Autodesk Inventor part; units mm, degrees
ref_plane "YZ Plane" through (0, 0, 0) normal (1, 0, 0) x (0, 1, 0)
ref_plane "XZ Plane" through (0, 0, 0) normal (0, 1, 0) x (-1, 0, 0)
ref_plane "XY Plane" through (0, 0, 0) normal (0, 0, 1) x (1, 0, 0)
sketch "Sketch_1" plane through (0, 0, 0) normal (0, 0, 1) x (1, 0, 0)
  line L0 (-57.15, 38.1) -> (-57.15, 0)
  line L1 (-57.15, 0) -> (57.15, 0)
  line L2 (57.15, 0) -> (57.15, 114.3)
  line L3 (57.15, 114.3) -> (19.05, 114.3)
  line L4 (19.05, 114.3) -> (-57.15, 38.1)
  circle A0 centre (38.1, 19.05) radius 4.1656
  circle A1 centre (38.1, 57.15) radius 4.1656
  circle A2 centre (38.1, 95.25) radius 4.1656
  circle A3 centre (0, 19.05) radius 4.1656
  circle A4 centre (0, 57.15) radius 4.1656
  circle A5 centre (-38.1, 19.05) radius 4.1656
extrude "Extrusion1" add sketch "Sketch_1" along normal mid plane 6.35
properties part number "4461"
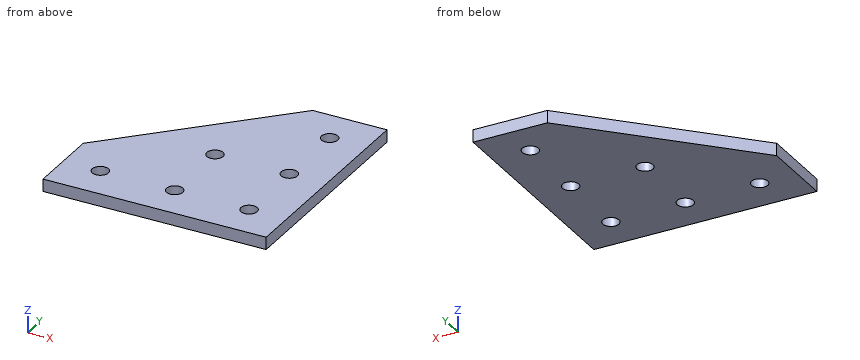
The model under review builds one solid part; all positions refer to its coordinate system, in mm. Coordinates: 2 decimals unless noted, no trailing zeros. Loops run counter-clockwise (first coordinate to the right, second up) from the corner with the lowest first, then second, coordinate; pieces in that order, holes last.
(1) Consider section C-C, the plane z = -1. Give the boundary of the cut face in (x, y).
Determined:
outline: (-57.15, 0) - (57.15, 0) - (57.15, 114.3) - (19.05, 114.3) - (-57.15, 38.1) - close; hole circle Ø8.33 at (-38.1, 19.05); hole circle Ø8.33 at (0, 19.05); hole circle Ø8.33 at (0, 57.15); hole circle Ø8.33 at (38.1, 19.05); hole circle Ø8.33 at (38.1, 57.15); hole circle Ø8.33 at (38.1, 95.25)
(2) Wall thickness on L1, parallel to Y at x = 38.1, z = -2; L2, parallel to X at y = 71, z = 0; L3, parallel to Y at x = 10, z = 2.5: over which ranges is each line inside the solid? List them lowest first.
Determined:
L1: y = 0 to 14.88, 23.22 to 52.98, 61.32 to 91.08, 99.42 to 114.3
L2: x = -24.25 to 57.15
L3: y = 0 to 105.25
(3) Consider section D-D, the plane x = -38.1. Give the boundary of the cut face in (y, z) (3 decimals).
Determined:
outline: (0, -3.175) - (14.884, -3.175) - (14.884, 3.175) - (0, 3.175) - close; (23.216, -3.175) - (57.15, -3.175) - (57.15, 3.175) - (23.216, 3.175) - close
(4) Insertion check: P1, Ø13.5, axis at x = -38.1, y = 19.05, coming from the -Z side (3 decimals); P2, Ø1, axis at y = 65.5, z = -2.5, coming from the -X side. Each pin has a flat end and moves straight along its axis. Give the tip position at first contact, or say it passes through.
Determined:
P1: stops at z = -3.175
P2: stops at x = -30.25
(5) Consider section A-A, the plane x = 0. Give the boundary of the cut face in (y, z) (3 decimals).
Determined:
outline: (0, -3.175) - (14.884, -3.175) - (14.884, 3.175) - (0, 3.175) - close; (23.216, -3.175) - (52.984, -3.175) - (52.984, 3.175) - (23.216, 3.175) - close; (61.316, -3.175) - (95.25, -3.175) - (95.25, 3.175) - (61.316, 3.175) - close
